Could you check a few things on this model? Use its own coordinates, in mm. Face numbers are marked on the shaded views. A direction names the side the tool comes from. Round coordinates to 2 decimals unless told otherwise and drop trailing zeros. Loops run counter-clockwise (first coordinate to the right, second up) from the corner with the lowest first, then second, coordinate; pieces in that order, holes last. Notation, with made-up numbers: (74.5, 59.25) - (112.5, 59.25) arc R37 ccw to (112.5, 98.25) - close; hole circle Ø3 at (15, 61.5). An arc over 180 degrees is marked (long way). Use one line per item in the form item = value.
```python
from build123d import *

# Parameters (mm, degrees)
EXTRUDE_1_DEPTH          = 15.25
CUT_EXTRUDE_1_DEPTH      = 26.550195694
CUT_EXTRUDE_1_DEPTH_BACK = 26.550195694
SKETCH_3_W               = 8.238165393
SKETCH_3_H               = 8.365
SKETCH_3_H_2             = 9.885
SKETCH_4_R               = 2
CUT_EXTRUDE_2_DEPTH      = 31.169657356
PATTERN_LINEAR_1_COUNT   = 2
PATTERN_LINEAR_1_PITCH   = 14


with BuildPart() as part:
    # 草图1 → 凸台-拉伸1 (new, symmetric)
    with BuildSketch(Plane.XY):
        with BuildLine():
            Line((17.464816242, 0), (4, 0))
            ThreePointArc((4, 0), (-2.371533507, 3.221153338), (-1.187914412, -3.819536536))
            Line((-1.187914412, -3.819536536), (1, -4.5))
            Line((1, -4.5), (20, -4.5))
            Line((20, -4.5), (20, -3.302775638))
            ThreePointArc((20, -3.302775638), (19.957092026, -3.012991489), (19.832050294, -2.748075442))
            Line((19.832050294, -2.748075442), (18.296866536, -0.445299804))
            ThreePointArc((18.296866536, -0.445299804), (17.936674167, -0.118325401), (17.464816242, 0))
        make_face()
    extrude(amount=EXTRUDE_1_DEPTH, both=True)

    # 草图3 → 切除-拉伸1 (cut, two sides: drawn at the far end of the back side and taken through both)
    with BuildSketch(Plane(origin=(0, 0, 0), x_dir=(1, 0, 0), z_dir=(0, 1, 0)).offset(-CUT_EXTRUDE_1_DEPTH_BACK)):
        with Locations((0.119082697, -11.0675)):
            Rectangle(SKETCH_3_W, SKETCH_3_H)
        with Locations((0.119082697, 3.9325)):
            Rectangle(SKETCH_3_W, SKETCH_3_H_2)
    extrude(amount=CUT_EXTRUDE_1_DEPTH + CUT_EXTRUDE_1_DEPTH_BACK, mode=Mode.SUBTRACT)

    # 草图4 → 切除-拉伸2 (cut, through all)
    with BuildSketch(Plane.XY.offset(6.885)):
        Circle(SKETCH_4_R)
    extrude(amount=-CUT_EXTRUDE_2_DEPTH, mode=Mode.SUBTRACT)

    # 草图5 → 切除-旋转1 (revolve, cut)
    with BuildSketch(Plane.XY.offset(7), mode=Mode.PRIVATE) as cut_revolve_1_sk:
        Polygon((10, -4.5), (10, 0), (14.4, 0), (14.4, -0.5), (12.5, -2), (12.5, -4.5), align=None)
    cut_revolve_1 = revolve(cut_revolve_1_sk.sketch.rotate(Axis((10, -4.5, 7), (0, 1, 0)), 90), axis=Axis((10, -4.5, 7), (0, 1, 0)), mode=Mode.SUBTRACT)

    # 阵列(线性)1: 切除-旋转1 ×2
    with Locations(*[(0, 0, -i * PATTERN_LINEAR_1_PITCH) for i in range(1, PATTERN_LINEAR_1_COUNT)]):
        add(cut_revolve_1, mode=Mode.SUBTRACT)


solid = part.part
```
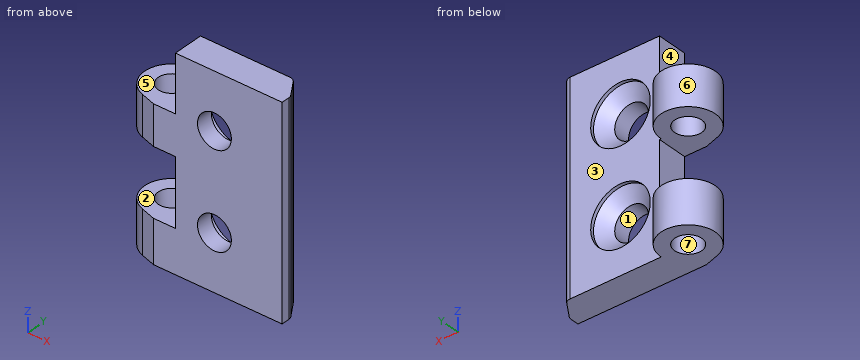
1. On a 3-axis mill with a long thin cutter (end or side, diameter ignored), from which of +Z, -Z, +X, -X, +Y, -Y can I reach the whole of each face in a straight line? I mean the marked faces 1, 2, 3 and 4. Say none if no direction works.
Solution:
face_1 = +Y, -Y
face_2 = -X, +Y, -Y
face_3 = +Z, -Z, +X, +Y
face_4 = +Z, -X, +Y, -Y
2. For P1, Ø5.5, axis at x = 10, z = 7, coming from the +Y side; P2, Ø3.5, axis at y = -2, z = -3, coming from the -X side; P3, Ø1.5, axis at x = 6.5, z = 2, coming from the +Y side, each with a flat end and sliding along its axis, tell me the tip position at first contact or that it passes through.
Solution:
P1 = -1.8
P2 = 4.24
P3 = 0
3. If we section it at D-D, the plane z = 0: Write out the boundary of the cut face in (x, y).
Solution:
outline = (4.24, -4.5) - (20, -4.5) - (20, -3.3) arc R1 ccw to (19.83, -2.75) - (18.3, -0.45) arc R1 ccw to (17.46, 0) - (4.24, 0) - close
4. If we section it at B-B, the plane y = -1.25: Write out the boundary of the cut face in (x, z) (3 decimals).
Solution:
outline = (-3.8, -15.25) - (-1.561, -15.25) - (-1.561, -8.875) - (-3.8, -8.875) - close; (-3.8, 1.01) - (-1.561, 1.01) - (-1.561, 6.885) - (-3.8, 6.885) - close; (1.561, -15.25) - (18.833, -15.25) - (18.833, 15.25) - (4.238, 15.25) - (4.238, 6.885) - (1.561, 6.885) - (1.561, 1.01) - (4.238, 1.01) - (4.238, -8.875) - (1.561, -8.875) - close; hole circle Ø6.9 at (10, -7); hole circle Ø6.9 at (10, 7)
5. Please list where these lines run through material, in increasing order: line 1 along Y through (x, z) = (9.5, -10.5); line 2 along Z through (x, y) = (11.5, -2.5); line 3 along X through (y, z) = (1.75, -13).
Solution:
line_1 = -4.5 to -1.18
line_2 = -15.25 to -9, -5 to 5, 9 to 15.25
line_3 = -3.6 to -0.97, 0.97 to 3.6
6. If we section it at C-C, the plane x = 10: Write out the boundary of the cut face in (y, z).
Solution:
outline = (-4.5, -15.25) - (0, -15.25) - (0, -11.4) - (-0.5, -11.4) - (-2, -9.5) - (-4.5, -9.5) - close; (-4.5, -4.5) - (-2, -4.5) - (-0.5, -2.6) - (0, -2.6) - (0, 2.6) - (-0.5, 2.6) - (-2, 4.5) - (-4.5, 4.5) - close; (-4.5, 9.5) - (-2, 9.5) - (-0.5, 11.4) - (0, 11.4) - (0, 15.25) - (-4.5, 15.25) - close
7. If we section it at A-A, the plane z = -7: Write out the boundary of the cut face in (x, y), plus the area to 3 significant figures.
Solution:
outline = (4.24, -4.5) - (7.5, -4.5) - (7.5, -2) - (5.6, -0.5) - (5.6, 0) - (4.24, 0) - close; (12.5, -4.5) - (20, -4.5) - (20, -3.3) arc R1 ccw to (19.83, -2.75) - (18.3, -0.45) arc R1 ccw to (17.46, 0) - (14.4, 0) - (14.4, -0.5) - (12.5, -2) - close
area = 40.6 mm^2
8. We'd pull the mould along Y, two halves only. Please class the marked faces 5, 6 and 7: +Y half, -Y half, draft (parallel to the pull), parting line (faces both ways), or undercut.
Solution:
face_5 = draft
face_6 = parting line
face_7 = undercut
